from build123d import *

# Parameters (mm, degrees)
SKETCH1_W                 = 55
SKETCH1_H                 = 20
MAIN_DEPTH                = 17.5
SKETCH3_W                 = 27
SKETCH3_H                 = 41.5
CENTRALHOLEFORSERVO_DEPTH = 21
SKETCH4_R                 = 1.25
FIXHOLESERVO_DEPTH        = 12
SKETCH5_R                 = 1.25
BOTTOMFIXHOLE_DEPTH       = 12
LPATTERN1_COUNT           = 4
LPATTERN1_PITCH           = 10
SKETCH6_W                 = 5
SKETCH6_H                 = 7
CUT_EXTRUDE4_DEPTH        = 27
SKETCH7_W                 = 1.75
SKETCH7_H                 = 7
CUT_EXTRUDE5_DEPTH        = 5


with BuildPart() as part:
    # Sketch1 → Main (new body, symmetric)
    with BuildSketch(Plane(origin=(0, 0, 0), x_dir=(0, 0, -1), z_dir=(1, 0, 0))):
        Rectangle(SKETCH1_W, SKETCH1_H)
    extrude(amount=MAIN_DEPTH, both=True)

    # Sketch3 → CentralHoleForServo (cut, through all)
    with BuildSketch(Plane(origin=(0, 10, 0), x_dir=(1, 0, 0), z_dir=(0, 1, 0))):
        with Locations((4, 0)):
            Rectangle(SKETCH3_W, SKETCH3_H)
    extrude(amount=-CENTRALHOLEFORSERVO_DEPTH, mode=Mode.SUBTRACT)

    # Sketch4 → FixHoleServo (cut)
    with BuildSketch(Plane(origin=(17.5, 0, 0), x_dir=(0, 0, -1), z_dir=(1, 0, 0))):
        with Locations((-24.5, 5)):
            Circle(SKETCH4_R)
        with Locations((-24.5, -5)):
            Circle(SKETCH4_R)
    fixholeservo = extrude(amount=-FIXHOLESERVO_DEPTH, mode=Mode.SUBTRACT)

    # FixHoleServoMirror: FixHoleServo across plane
    add(fixholeservo.mirror(Plane.XY), mode=Mode.SUBTRACT)

    # Sketch5 → BottomFixHole (cut)
    with BuildSketch(Plane.ZY.offset(17.5)):
        with Locations((15, 5)):
            Circle(SKETCH5_R)
        with Locations((15, -5)):
            Circle(SKETCH5_R)
    bottomfixhole = extrude(amount=-BOTTOMFIXHOLE_DEPTH, mode=Mode.SUBTRACT)

    # LPattern1: BottomFixHole ×4
    with Locations(*[(0, 0, -i * LPATTERN1_PITCH) for i in range(1, LPATTERN1_COUNT)]):
        add(bottomfixhole, mode=Mode.SUBTRACT)

    # Sketch6 → Cut-Extrude4 (cut)
    with BuildSketch(Plane(origin=(17.5, 0, 0), x_dir=(0, 0, -1), z_dir=(1, 0, 0))):
        with Locations((-23.25, 0)):
            Rectangle(SKETCH6_W, SKETCH6_H)
    extrude(amount=-CUT_EXTRUDE4_DEPTH, mode=Mode.SUBTRACT)

    # Sketch7 → Cut-Extrude5 (cut)
    with BuildSketch(Plane(origin=(17.5, 0, 0), x_dir=(0, 0, -1), z_dir=(1, 0, 0))):
        with Locations((-26.625, 0)):
            Rectangle(SKETCH7_W, SKETCH7_H)
    extrude(amount=-CUT_EXTRUDE5_DEPTH, mode=Mode.SUBTRACT)


solid = part.part
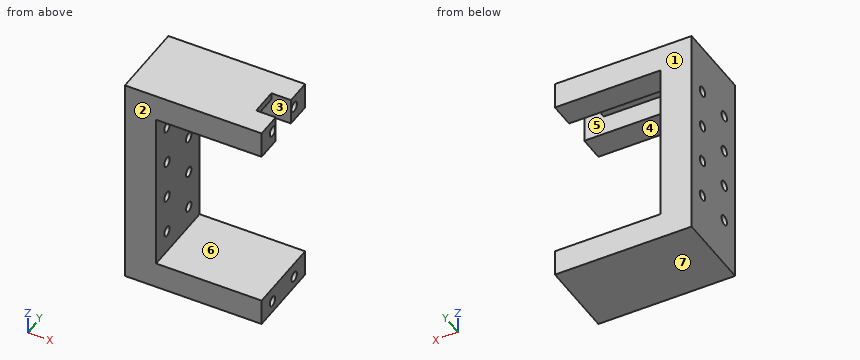
Source: CAD feature listing. Evaluate the final solid. Frame: model axes, mm. Face numbers are marked on the shaded views. A direction names the side the tool comes from. Round coordinates to 2 decimals unless told otherwise and drop trailing zeros. Loops run counter-clockwise (first coordinate to the right, second up) from the corner with the lowest first, then second, coordinate; pieces in that order, holes last.
Q1. Section B-B, the plane y = -5. State how many separate pieces and enclosed holes the cut face has, plus the area to 4 significant figures.
Q2. Section A-A, the plane z = 5. Return loops of the section in (x, y), plus the area to 3 significant figures.
Q3. Section D-D, the plane x = 2.5. Return loops of the section in (y, z).
Q4. Mould query, pull axis Y, two halves, no side actions, for the marked faces 1, 2, 3 and 4. Classes: pulls with the +Y half, pulls with the -Y half, needs draft (parallel to the pull), parting line crosses it, or undercut.
Q5. Section C-C, the plane x = 13.5. Return loops of the section in (y, z).
Q6. Access query for the marked faces 5, 6 and 7. Directions: +Z, -Z, +X, -X, +Y, -Y. A direction counts if a zero-diameter tool reaches every point of the face in a straight line with its end or side. Return the directions, or none.
Q7. Ray query, line 1 (Y direction, x = 14.75, z = 24.5); line 2 (Y direction, x = 14.5, z = -24.5); line 3 (Z direction, x = 4.5, y = 4.25). Return the intervals inside material, ascending.
Q8. First-contact query: P1, Ø1.2, axis at y = 5.5, z = 24.5, coming from the +X side; P2, Ø1.5, axis at y = -5, z = 5, coming from the -X side; P3, Ø6, axis at y = 4, z = -10, coming from the +X side. Flat tips, straight axial feed; report the tip coordinate or a pass-through.
Solutions:
1. separate pieces: 5
1. enclosed holes: 0
1. area: 664.5 mm2
2. outline: (-17.5, -10) - (-9.5, -10) - (-9.5, -6.25) - (-17.5, -6.25) - close; (-17.5, -3.75) - (-9.5, -3.75) - (-9.5, 3.75) - (-17.5, 3.75) - close; (-17.5, 6.25) - (-9.5, 6.25) - (-9.5, 10) - (-17.5, 10) - close
2. area: 120 mm2
3. outline: (-10, -27.5) - (10, -27.5) - (10, -20.75) - (-10, -20.75) - close; (-10, 20.75) - (-3.5, 20.75) - (-3.5, 25.75) - (3.5, 25.75) - (3.5, 20.75) - (10, 20.75) - (10, 27.5) - (-10, 27.5) - close
4. face 1: pulls with the +Y half
4. face 2: pulls with the -Y half
4. face 3: undercut
4. face 4: needs draft
5. outline: (-10, -27.5) - (10, -27.5) - (10, -20.75) - (-10, -20.75) - close; (-10, 20.75) - (-3.5, 20.75) - (-3.5, 27.5) - (-10, 27.5) - close; (3.5, 20.75) - (10, 20.75) - (10, 27.5) - (3.5, 27.5) - close; hole circle Ø2.5 at (-5, -24.5); hole circle Ø2.5 at (-5, 24.5); hole circle Ø2.5 at (5, -24.5); hole circle Ø2.5 at (5, 24.5)
6. face 5: +X
6. face 6: +X, +Y, -Y
6. face 7: -Z, +X, -X, +Y, -Y
7. line 1: y = -10 to -6.25, -3.75 to -3.5, 3.5 to 3.75, 6.25 to 10
7. line 2: y = -10 to -6.25, -3.75 to 3.75, 6.25 to 10
7. line 3: z = -27.5 to -20.75, 20.75 to 27.5
8. P1: stops at x = 5.5
8. P2: passes through
8. P3: stops at x = -9.5
